Source: CAD feature listing. Evaluate the final solid. Frame: model axes, mm. A direction names the side the tool comes from. Round coordinates to 2 decimals unless told otherwise and drop trailing zeros. Write each loop counter-clockwise with the first axis right and the second up, starting at its lowest first coordinate (ties: lowest second). Pieces come first, ordered by that corner, then holes.
from build123d import *

# Parameters (mm, degrees)
SKETCH1_W           = 10
SKETCH1_H           = 25
SKETCH1_R           = 2.1
BOSS_EXTRUDE1_DEPTH = 7
SKETCH2_W           = 10
SKETCH2_H           = 8
BOSS_EXTRUDE2_DEPTH = 12
SKETCH3_R           = 1.7
CUT_EXTRUDE1_DEPTH  = 33.954514107
SKETCH4_R           = 3
CUT_EXTRUDE2_DEPTH  = 4


with BuildPart() as part:
    # Sketch1 → Boss-Extrude1 (new body)
    with BuildSketch(Plane(origin=(0, 0, 0), x_dir=(1, 0, 0), z_dir=(0, 1, 0))):
        with Locations((5, 12.5)):
            Rectangle(SKETCH1_W, SKETCH1_H)
        with Locations(Location((5, 21, 0), (0, 0, 270))):
            Circle(SKETCH1_R, mode=Mode.SUBTRACT)
    extrude(amount=BOSS_EXTRUDE1_DEPTH)

    # Sketch2 → Boss-Extrude2 (add)
    with BuildSketch(Plane(origin=(0, 0, 0), x_dir=(-1, 0, 0), z_dir=(0, -1, 0))):
        with Locations((-5, 4)):
            Rectangle(SKETCH2_W, SKETCH2_H)
    extrude(amount=BOSS_EXTRUDE2_DEPTH)

    # Sketch3 → Cut-Extrude1 (cut, through all)
    with BuildSketch(Plane(origin=(0, 7, 0), x_dir=(1, 0, 0), z_dir=(0, 1, 0))):
        with Locations(Location((5, 4.25, 0), (0, 0, 270))):
            Circle(SKETCH3_R)
    extrude(amount=-CUT_EXTRUDE1_DEPTH, mode=Mode.SUBTRACT)

    # Sketch4 → Cut-Extrude2 (cut)
    with BuildSketch(Plane(origin=(0, 7, 0), x_dir=(1, 0, 0), z_dir=(0, 1, 0))):
        with Locations(Location((5, 4.25, 0), (0, 0, 270))):
            Circle(SKETCH4_R)
    extrude(amount=-CUT_EXTRUDE2_DEPTH, mode=Mode.SUBTRACT)


solid = part.part
1) Contact query for flat-ended pins moving along their axis: P1, Ø4, axis at x = 1.5, z = -19, coming from the -Y side; P2, Ø1.8, axis at x = 6.5, z = -3.5, coming from the +Y side. Output: stop coordinate, or through.
Taken from the geometry:
P1: stops at y = 0
P2: stops at y = 3
2) Section query C-C on y = 3.5. Return the cut outline in (x, z).
Taken from the geometry:
outline: (0, -25) - (10, -25) - (10, 0) - (0, 0) - close; hole circle Ø6 at (5, -4.25); hole circle Ø4.2 at (5, -21)
3) Pull-direction query (Z, two-part tool) for faces 3 (the face through (5, -6, -8)), 4 (the face through (10, 2, -10)), 5 (the face through (2.338, 5.028, -2.866)), 6 (the face through (3, 3, -4)); classes: released by +Z, released by -Z, zero draft, split by the parting line, or undercut.
Taken from the geometry:
face 3: released by -Z
face 4: zero draft
face 5: undercut
face 6: undercut
4) Section query B-B on z = -4.25. Return the cut outline in (x, y), then the cut area to 3 significant figures.
Taken from the geometry:
outline: (0, -12) - (3.3, -12) - (3.3, 3) - (2, 3) - (2, 7) - (0, 7) - close; (6.7, -12) - (10, -12) - (10, 7) - (8, 7) - (8, 3) - (6.7, 3) - close
area: 115 mm2
5) Reachability of faces 1 (the face through (5, 0, -17)), 2 (the face through (5, -2, 0)) from +Z, -Z, +X, -X, +Y, -Y: full face, straight path, thin tool, end or side. Return the list, or none.
Taken from the geometry:
face 1: -Z, +X, -X, -Y
face 2: +Z, +X, -X, +Y, -Y
6) Section query A-A on x = 5. Return the cut outline in (y, z), then the cut area to 3 significant figures.
Taken from the geometry:
outline: (-12, -8) - (0, -8) - (0, -18.9) - (7, -18.9) - (7, -7.25) - (3, -7.25) - (3, -5.95) - (-12, -5.95) - close; (-12, -2.55) - (3, -2.55) - (3, -1.25) - (7, -1.25) - (7, 0) - (-12, 0) - close; (0, -25) - (7, -25) - (7, -23.1) - (0, -23.1) - close
area: 167 mm2
7) Material intervals for line 1 (Z direction, x = 5.75, y = 0.5); line 2 (X direction, y = 5.3, z = -4.25); line 3 (Y direction, x = 7.25, z = -18.25), sorted ascending.
Taken from the geometry:
line 1: z = -25 to -22.96, -19.04 to -5.78, -2.72 to 0
line 2: x = 0 to 2, 8 to 10
line 3: y = 0 to 7
8) Section query D-D on y = -5.5. Return the cut outline in (x, z).
Taken from the geometry:
outline: (0, -8) - (10, -8) - (10, 0) - (0, 0) - close; hole circle Ø3.4 at (5, -4.25)
